Could you check a few things on this drawing? It's one solid part, dimensions in mm from its lowest x, y, z. A direction names the side the tool comes from. Round coordinates to 2 decimals unless told otherwise and drop trailing zeros. Write each loop counter-clockwise with the first axis right and the second up, starting at its lowest first coordinate (ties: lowest second). Pieces come first, ordered by that corner, then holes. Notation, with made-up numbers: M -20.75,16.5 L 20.25,16.5 A22 cw 20.25,25.5 Z; hole C 88,-24.5 d2. An arc over 180 degrees is marked long. One line per item, written item: value. Start each with the question number.
(1) Which directions (+Z, -Z, +X, -X, +Y, -Y) give clear straight access to the entire face, cutting with the end or side of a thin tool? Please do the marked faces 1, 2, 3 and 4.
(2) I want a section at B-B on x = 7.25. Please give me the cut outline in (y, z) (1 decimal).
(3) I want a section at A-A on y = 12.5. Please give me the cut outline in (x, z).
(4) I want a section at C-C on x = 14.5. Please give me the cut outline in (y, z).
(5) I'm going to push flat-ended pins straight in: pin 1 Ø1.5 at (x, z) = (3.5, 3.5) entering from -Y; pin 2 Ø2 at (x, y) = (11, 15) entering from +Z; pin 3 Ø2 at (x, y) = (10.5, 3.5) entering from +Z (1 decimal); pin 4 Ø4.5 at (x, y) = (1, 10) entering from +Z. Where does each tip first touch, or does it pass through?
(6) If I drill on L1, parallel to X at y = 1.25, z = 4.25; L2, parallel to X at y = 8, z = 0.5; L3, parallel to Y at x = 14, z = 3.75, over which ranges is the centre line in solid material (lowest first)?
(7) Thinking about a two-plate mould opening in X: for the marked faces 5, 6, 7 and 8, which applies, released by +X, released by -X, zero draft, split by the parting line, or undercut?
(8) I want a section at D-D on z = 6.5. Please give me the cut outline in (x, y).
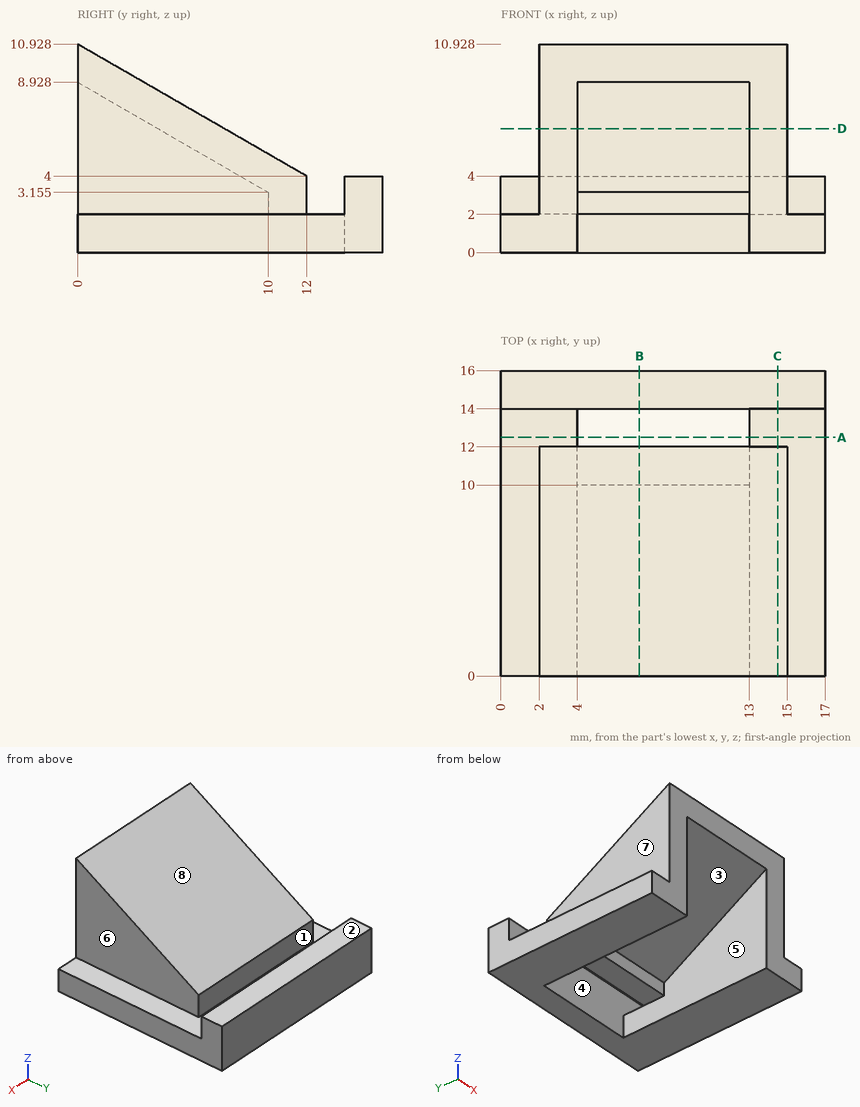
Found:
1. face 1: +Z, +X, -X
1. face 2: +Z, +X, -X, +Y
1. face 3: -Z, -Y
1. face 4: +Z
2. outline: M 0,8.9 L 10,3.2 L 10,2 L 12,2 L 12,4 L 0,10.9 Z; M 14,0 L 16,0 L 16,4 L 14,4 Z
3. outline: M 0,0 L 4,0 L 4,2 L 0,2 Z; M 13,0 L 17,0 L 17,2 L 13,2 Z
4. outline: M 0,0 L 16,0 L 16,4 L 14,4 L 14,2 L 12,2 L 12,4 L 0,10.93 Z
5. pin 1: stops at y = 0
5. pin 2: stops at z = 4
5. pin 3: stops at z = 9.5
5. pin 4: stops at z = 6.32
6. L1: x = 2 to 4, 13 to 15
6. L2: x = 0 to 4, 13 to 17
6. L3: y = 0 to 12, 14 to 16
7. face 5: undercut
7. face 6: released by +X
7. face 7: released by -X
7. face 8: zero draft
8. outline: M 2,0 L 4,0 L 4,4.21 L 13,4.21 L 13,0 L 15,0 L 15,7.67 L 2,7.67 Z
